from build123d import *

# Parameters (mm, degrees)
SKETCH1_W           = 31
SKETCH1_H           = 30
SKETCH1_R           = 1.2
SKETCH1_W_2         = 21.4
SKETCH1_H_2         = 8.3
BOSS_EXTRUDE1_DEPTH = 4
SKETCH1_6_R         = 2.8
SKETCH1_6_R_2       = 1.2
CUT_EXTRUDE1_DEPTH  = 2
FILLET1_R           = 6


with BuildPart() as part:
    # Sketch1 → Boss-Extrude1 (new body)
    with BuildSketch(Plane.XY):
        Rectangle(SKETCH1_W, SKETCH1_H)
        with Locations((-10.7, 9.8)):
            Circle(SKETCH1_R, mode=Mode.SUBTRACT)
        with Locations((10.7, 9.8)):
            Circle(SKETCH1_R, mode=Mode.SUBTRACT)
        with Locations((10.7, -4.5)):
            Circle(SKETCH1_R, mode=Mode.SUBTRACT)
        with Locations((-10.7, -4.5)):
            Circle(SKETCH1_R, mode=Mode.SUBTRACT)
        with Locations((-7.5, -11)):
            Circle(SKETCH1_R, mode=Mode.SUBTRACT)
        with Locations((7.5, -11)):
            Circle(SKETCH1_R, mode=Mode.SUBTRACT)
        with Locations((0, 2.65)):
            Rectangle(SKETCH1_W_2, SKETCH1_H_2, mode=Mode.SUBTRACT)
    extrude(amount=BOSS_EXTRUDE1_DEPTH)

    # Sketch1<6> → Cut-Extrude1 (cut)
    # profile 1 of 2: a face of its own
    with BuildSketch(Plane.XY):
        with Locations((-7.5, -11)):
            Circle(SKETCH1_6_R)
        with Locations((-7.5, -11)):
            Circle(SKETCH1_6_R_2, mode=Mode.SUBTRACT)
    # profile 2 of 2: a face of its own
    with BuildSketch(Plane.XY):
        with Locations((7.5, -11)):
            Circle(SKETCH1_6_R)
        with Locations((7.5, -11)):
            Circle(SKETCH1_6_R_2, mode=Mode.SUBTRACT)
    extrude(amount=CUT_EXTRUDE1_DEPTH, mode=Mode.SUBTRACT)

    # Fillet1
    fillet1_edges = [part.edges().sort_by_distance(p)[0] for p in [
        (-15.5, -15, 2),
        (-15.5, 15, 2),
        (15.5, 15, 2),
        (15.5, -15, 2),
    ]]
    fillet(fillet1_edges, radius=FILLET1_R)


solid = part.part
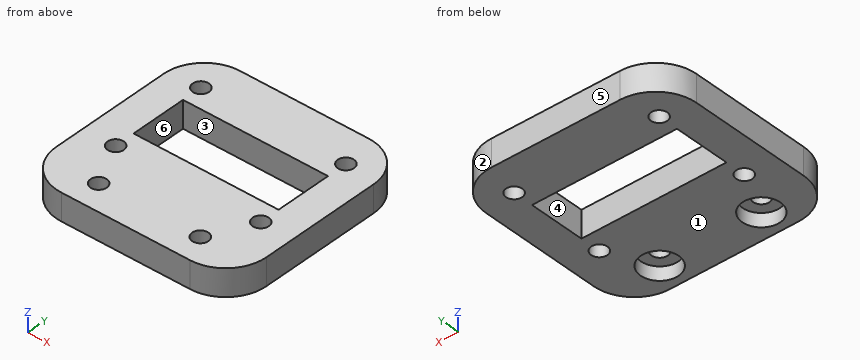
Geometry check sheet. Reference: the model listing, model coordinates, mm. Face numbers are marked on the shaded views. A direction names the side the tool comes from. Coordinates: 2 decimals unless noted, no trailing zeros. Order: outer loops, then holes, each group sorted by start corner. A loop starts at its lowest first (then second) coordinate and runs counter-clockwise, first axis right, second up. Notation, with made-up numbers: (38.25, 22) - (44.25, 22) arc R21 cw to (44.25, 37) - close; hole circle Ø5 at (56, 63). An arc over 180 degrees is marked (long way). Answer in a Markdown table with one row per item. Add a question column.
1) Cross-section at B-B, the plane y = -4.5. Record the cut outline in (x, z), then the cut area to 3 significant figures.
2) Gauge pin test, flat ends, axial feed: P1, Ø5, axis at x = -7.5, y = -11, coming from the -Z side; P2, Ø1.9, axis at x = 7.5, y = -11, coming from the +Z side. Record the tip position at first contact, or that the pin passes through.
3) Material ranges on line 1 along Y through (x, z) = (7.5, 3.35); line 2 along Y through (x, z) = (6, 3.2); line 3 along Y through (x, z) = (-11.5, 1.25), recorded low to high. Write a range as [from, to].
4) Release check for a two-part mould opening along X. For the marked faces 1, 2, 3 and 4 record: +X half, -X half, draft (parallel to the pull), parting line (faces both ways), or undercut.
5) Cross-section at D-D, the plane z = 1.2. Record the cut outline in (x, y).
6) Cross-section at A-A, the plane x = -7.5. Record the cut outline in (y, z), then the cut area to 3 significant figures.
7) Set-up check for the marked faces 5 and 6: record each of +Z, -Z, +X, -X, +Y, -Y from which the full face is reachable in a straight line by a thin tool's end or side.
8) Cross-section at C-C, the plane x = 3. Record the cut outline in (y, z), then the cut area to 3 significant figures.
Check result:
| question | item | result |
|---|---|---|
| 1 | outline | (-15.5, 0) - (-11.9, 0) - (-11.9, 4) - (-15.5, 4) - close; (-9.5, 0) - (9.5, 0) - (9.5, 4) - (-9.5, 4) - close; (11.9, 0) - (15.5, 0) - (15.5, 4) - (11.9, 4) - close |
| 1 | area | 105 mm² |
| 2 | P1 | stops at z = 2 |
| 2 | P2 | passes through |
| 3 | line 1 | y = [-15, -12.2], [-9.8, -1.5], [6.8, 15] |
| 3 | line 2 | y = [-15, -1.5], [6.8, 15] |
| 3 | line 3 | y = [-14.66, -5.39], [-3.61, 8.91], [10.69, 14.66] |
| 4 | face 1 | draft |
| 4 | face 2 | +X half |
| 4 | face 3 | undercut |
| 4 | face 4 | undercut |
| 5 | outline | (-15.5, -9) arc R6 ccw to (-9.5, -15) - (9.5, -15) arc R6 ccw to (15.5, -9) - (15.5, 9) arc R6 ccw to (9.5, 15) - (-9.5, 15) arc R6 ccw to (-15.5, 9) - close; hole circle Ø2.4 at (-10.7, -4.5); hole circle Ø2.4 at (-10.7, 9.8); hole (-10.7, -1.5) - (10.7, -1.5) - (10.7, 6.8) - (-10.7, 6.8) - close; hole circle Ø5.6 at (-7.5, -11); hole circle Ø5.6 at (7.5, -11); hole circle Ø2.4 at (10.7, -4.5); hole circle Ø2.4 at (10.7, 9.8) |
| 6 | outline | (-15, 0) - (-13.8, 0) - (-13.8, 2) - (-12.2, 2) - (-12.2, 4) - (-15, 4) - close; (-9.8, 2) - (-8.2, 2) - (-8.2, 0) - (-1.5, 0) - (-1.5, 4) - (-9.8, 4) - close; (6.8, 0) - (15, 0) - (15, 4) - (6.8, 4) - close |
| 6 | area | 70.8 mm² |
| 7 | face 5 | +Z, -Z, +X, -X, +Y |
| 7 | face 6 | +Z, -Z |
| 8 | outline | (-15, 0) - (-1.5, 0) - (-1.5, 4) - (-15, 4) - close; (6.8, 0) - (15, 0) - (15, 4) - (6.8, 4) - close |
| 8 | area | 86.8 mm² |
